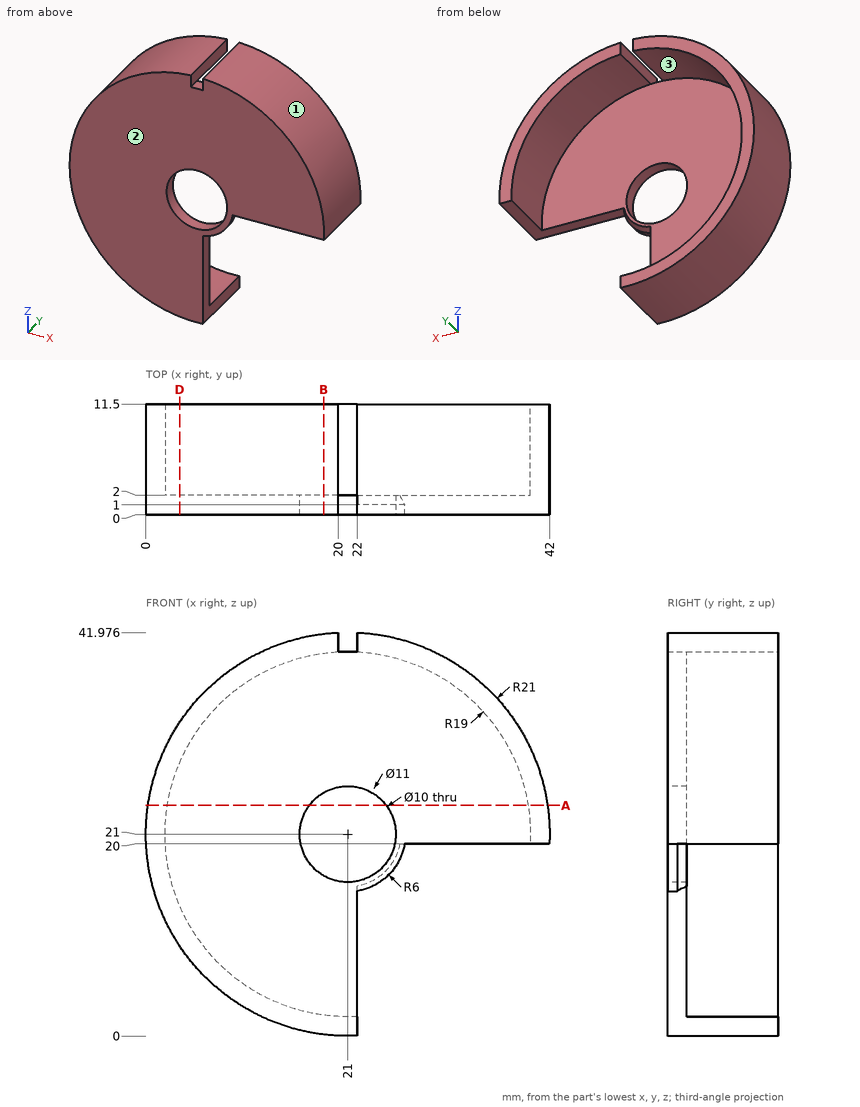
Can you work these out from the drawing? Everything is in mm from the part's minimum corner. Round coordinates to 2 decimals unless told otherwise and drop trailing zeros. Loops run counter-clockwise (first coordinate to the right, second up) from the corner with the lowest first, then second, coordinate; pieces in that order, holes last.
1. We'd pull the mould along X, two halves only. Please class the marked faces 1, 2 and 3: +X half, -X half, draft (parallel to the pull), parting line (faces both ways), or undercut.
Answer list:
face 1: +X half
face 2: draft
face 3: undercut
2. For P1, Ø3, axis at y = 9.5, z = 12.5, coming from the -X side; P2, Ø4, axis at y = 4.5, z = 14, coming from the +X side; P3, Ø1.5, axis at x = 6, y = 10, coming from the +Z side (1 decimal), each with a flat end and sliding along its axis, tell me the tip position at first contact or that it passes through.
Answer list:
P1: stops at x = 1.2
P2: stops at x = 4.27
P3: stops at z = 36.4
3. If I drill on line 1 along Z through (x, y) = (21, 1); line 2 along Z through (x, y) = (14, 2.5); line 3 along X through (y, z) = (9.5, 20.5), over which ranges is the centre line in solid material (lowest first)?
Answer list:
line 1: z = 0 to 16, 26 to 40
line 2: z = 1.2 to 3.34, 38.66 to 40.8
line 3: x = 0.01 to 2.01, 39.99 to 41.99
4. If we section it at A-A on z = 24: Write out the boundary of the cut face in (x, y) (1 decimal).
Answer list:
outline: (0.2, 0) - (17, 0) - (17, 2) - (2.2, 2) - (2.2, 11.5) - (0.2, 11.5) - close; (25, 0) - (41.8, 0) - (41.8, 11.5) - (39.8, 11.5) - (39.8, 2) - (25, 2) - close
5. If we section it at D-D on x = 3.5: Write out the boundary of the cut face in (y, z), plus the area to 3 significant figures.
Answer list:
outline: (0, 9.39) - (11.5, 9.39) - (11.5, 13.6) - (2, 13.6) - (2, 28.4) - (11.5, 28.4) - (11.5, 32.61) - (0, 32.61) - close
area: 126 mm2
6. If we section it at B-B on x = 18.5: Write out the boundary of the cut face in (y, z) (1 decimal).
Answer list:
outline: (0, 0.1) - (11.5, 0.1) - (11.5, 2.2) - (2, 2.2) - (2, 16.7) - (0, 16.7) - close; (0, 25.3) - (2, 25.3) - (2, 39.8) - (11.5, 39.8) - (11.5, 41.9) - (0, 41.9) - close
